Work out the finished part from the listing and answer in its coordinate system (mm). A direction names the side the tool comes from. Give positions to 0.01 mm unless a question says otherwise; leave off trailing zeros. Loops run counter-clockwise (first coordinate to the right, second up) from the corner with the lowest first, then second, coordinate; pieces in that order, holes last. Notation, with made-up numbers: M 69,14 L 73,14 A28 ccw 73,32 Z; hole C 23.5,68.5 d8. An arc over 180 degrees is marked long. Write item = value, one per line. Start each with the question number.
1. Section A-A on z = 12 is taken. Determine the outline of the cut face in (x, y).
2. The mould has two halves that part along Z. Classify faces 3 (the face through (0, 31, -15)), 4 (the face through (2.3, 16, 0)), 5 (the face through (-0.042, 3.845, -12.921)), 6 (the face through (0, 31, 15)): released by +Z, released by -Z, zero draft, split by the parting line, or undercut.
3. Consider L1, parallel to Y at x = 1.25, z = 12; L2, parallel to Z at x = 0, y = 59; L3, parallel to Y at x = 2.7, z = -4.5. Determine where each line is inside the solid, lowest interval first. Write a range as [from, to].
4. Section B-B on y = 3 is taken. Determine the outline of the cut face in (x, z), plus the area to 3 significant figures.
5. Section C-C on y = 52.5 is taken. Determine the outline of the cut face in (x, z), plus the area to 3 significant figures.
6. Section D-D on y = 19 is taken. Determine the outline of the cut face in (x, z), plus the area to 3 significant figures.
7. For faces 1 (the face through (-0.042, 28.845, -12.921)), 2 (the face through (1.216, 56.879, -8.615)), determine the directions among +Z, -Z, +X, -X, +Y, -Y from which every point of the face is accessible in a straight line to the end or side of a thin tool.
```python
from build123d import *

# Parameters (mm, degrees)
SKETCH_1_W             = 6
SKETCH_1_H             = 30
EXTRUDE_1_DEPTH        = 62
HOLE_WIZARD_M4_1_D     = 3.3
HOLE_WIZARD_M4_1_DEPTH = 10.1
HOLE_WIZARD_M4_1_TIP   = 0.991420021
SKETCH_4_W             = 30
SKETCH_4_H             = 22
CUT_EXTRUDE_1_DEPTH    = 0.7
HOLE_WIZARD_M3_1_D     = 2.5


with BuildPart() as part:
    # 草图1 → 凸台-拉伸1 (new body)
    with BuildSketch(Plane(origin=(0, 0, 0), x_dir=(1, 0, 0), z_dir=(0, 1, 0))):
        Rectangle(SKETCH_1_W, SKETCH_1_H)
    extrude(amount=EXTRUDE_1_DEPTH)

    # M4 螺纹孔1
    with Locations(Plane(origin=(0, 62, 0), x_dir=(1, 0, 0), z_dir=(0, 1, 0))):
        with Locations((0, 7.5), (0, -7.5)):
            Hole(HOLE_WIZARD_M4_1_D / 2, depth=HOLE_WIZARD_M4_1_DEPTH)
            with Locations((0, 0, -(HOLE_WIZARD_M4_1_DEPTH + HOLE_WIZARD_M4_1_TIP / 2))):  # 118° drill point
                Cone(0, HOLE_WIZARD_M4_1_D / 2, HOLE_WIZARD_M4_1_TIP, mode=Mode.SUBTRACT)

    # 草图4 → 切除-拉伸1 (cut)
    with BuildSketch(Plane(origin=(3, 0, 0), x_dir=(0, 0, -1), z_dir=(1, 0, 0))):
        with Locations((0, 15.5)):
            Rectangle(SKETCH_4_W, SKETCH_4_H)
    extrude(amount=-CUT_EXTRUDE_1_DEPTH, mode=Mode.SUBTRACT)

    # M3 螺纹孔1 (through all)
    with Locations(Plane(origin=(3, 0, 0), x_dir=(0, 0, -1), z_dir=(1, 0, 0))):
        with Locations((-12, 28), (12, 28), (12, 3), (-12, 3)):
            Hole(HOLE_WIZARD_M3_1_D / 2)


solid = part.part
```
Verdict:
q1.outline = M -3,0 L 3,0 L 3,1.75 L -3,1.75 Z; M -3,4.25 L 3,4.25 L 3,4.5 L 2.3,4.5 L 2.3,26.5 L 3,26.5 L 3,26.75 L -3,26.75 Z; M -3,29.25 L 3,29.25 L 3,62 L -3,62 Z
q2.face_3 = released by -Z
q2.face_4 = zero draft
q2.face_5 = undercut
q2.face_6 = released by +Z
q3.L1 = [0, 1.75], [4.25, 26.75], [29.25, 62]
q3.L2 = [-15, -9.15], [-5.85, 5.85], [9.15, 15]
q3.L3 = [0, 4.5], [26.5, 62]
q4.outline = M -3,-15 L 3,-15 L 3,-13.25 L -3,-13.25 Z; M -3,-10.75 L 3,-10.75 L 3,10.75 L -3,10.75 Z; M -3,13.25 L 3,13.25 L 3,15 L -3,15 Z
q4.area = 150 mm2
q5.outline = M -3,-15 L 3,-15 L 3,15 L -3,15 Z; hole C 0,-7.5 d3.3; hole C 0,7.5 d3.3
q5.area = 163 mm2
q6.outline = M -3,-15 L 2.3,-15 L 2.3,15 L -3,15 Z
q6.area = 159 mm2
q7.face_1 = +X, -X
q7.face_2 = +Y
